Model file for the job. Use its own axes, mm. A direction names the side the tool comes from. Round coordinates to 2 decimals unless told otherwise and drop trailing zeros. Loops run counter-clockwise (first coordinate to the right, second up) from the corner with the lowest first, then second, coordinate; pieces in that order, holes last. Notation, with made-up numbers: (27, 59) -> (83, 59) arc R6 cw to (83, 67) -> close; hole circle Ø9 at (10.25, 39). An arc over 180 degrees is marked (long way). Use a Markdown table: item, result.
from build123d import *

# Parameters (mm, degrees)
F0_W      = 30
F0_H      = 22
F1_DEPTH  = 72
F3_DEPTH  = 72.001
F4_DEPTH  = 7
F6_DEPTH  = 7
F7_W      = 8
F7_H      = 44
F8_DEPTH  = 30.001
F9_W      = 30
F9_H      = 7
F10_DEPTH = 60
F11_R     = 4
F12_DEPTH = 65.001


with BuildPart() as f1:
    # F0 (on Top) → F1 (new body)
    with BuildSketch(Plane.XY):
        with Locations((15, 11)):
            Rectangle(F0_W, F0_H)
        Polygon((0, 102), (0, 22), (30, 22), (6.9943696583, 102.2807010551), align=None)
    extrude(amount=F1_DEPTH)

    # F2 (on face) → F3 (cut, through all)
    with BuildSketch(Plane.XY.offset(72)):
        Polygon((7, 22), (30, 22), (6.9943696583, 102.2807010551), align=None)
    extrude(amount=-F3_DEPTH, mode=Mode.SUBTRACT)

    # F2 (on face) → F4 (join)
    with BuildSketch(Plane.XY.offset(72)):
        Polygon((7, 22), (30, 22), (6.9943696583, 102.2807010551), align=None)
    extrude(amount=-F4_DEPTH)

    # F5 (on face) → F6 (join)
    with BuildSketch(Plane(origin=(0, 0, 0), x_dir=(1, 0, 0), z_dir=(0, 0, -1))):
        Polygon((6.9943696583, -102.2807010551), (30, -22), (7, -22), align=None)
    extrude(amount=-F6_DEPTH)

    # F7 (on face) → F8 (cut, through all)
    with BuildSketch(Plane.YZ.offset(30)):
        Polygon((16, 65), (8, 65), (8, 58), (8, 14), (8, 7), (16, 7), align=None)
        with Locations((4, 36)):
            Rectangle(F7_W, F7_H)
    extrude(amount=-F8_DEPTH, mode=Mode.SUBTRACT)

    # F9 (on face) → F10 (join)
    with BuildSketch(Plane.XZ):
        with Locations((15, 61.5)):
            Rectangle(F9_W, F9_H)
    extrude(amount=F10_DEPTH)

    # F11 (on face) → F12 (cut, through all)
    with BuildSketch(Plane.XY.offset(65)):
        with Locations((15, -44)):
            Circle(F11_R)
    extrude(amount=-F12_DEPTH, mode=Mode.SUBTRACT)


solid = f1.part
Q1. Band-saw the part on B-B, the plane x = 12.5. Give the cut face in (y, z), plus the area to 3 significant figures.
Results list:
| item | result |
|---|---|
| outline | (-60, 58) -> (-47.12, 58) -> (-47.12, 65) -> (-60, 65) -> close; (-40.88, 58) -> (8, 58) -> (8, 65) -> (16, 65) -> (16, 7) -> (8, 7) -> (8, 14) -> (0, 14) -> (0, 0) -> (83.07, 0) -> (83.07, 7) -> (22, 7) -> (22, 65) -> (83.07, 65) -> (83.07, 72) -> (0, 72) -> (0, 65) -> (-40.88, 65) -> close |
| area | 2,000 mm² |
Q2. Band-saw the part on D-D, the plane y = -44. Give the cut face in (x, z).
Results list:
| item | result |
|---|---|
| outline | (0, 58) -> (11, 58) -> (11, 65) -> (0, 65) -> close; (19, 58) -> (30, 58) -> (30, 65) -> (19, 65) -> close |
Q3. Band-saw the part on C-C, the plane z = 37. Give the cut face in (x, y), plus the area to 3 significant figures.
Results list:
| item | result |
|---|---|
| outline | (0, 16) -> (30, 16) -> (30, 22) -> (7, 22) -> (6.99, 102.28) -> (0, 102) -> close |
| area | 741 mm² |
Q4. Tool access for faces 1 (the face through (15, 4, 14)), 2 (the face through (15, -30, 65)), 3 (the face through (16, 53, 7)), 4 (the face through (15, 16, 36)): list every direction of +Z, -Z, +X, -X, +Y, -Y with a clear straight run to the whole face (end or side of a thin tool).
Results list:
| item | result |
|---|---|
| face 1 | +X, -X, -Y |
| face 2 | +Z, +X, -X, -Y |
| face 3 | +X, +Y |
| face 4 | +X, -X |
Q5. Band-saw the part on A-A, the plane y = 10. Give the cut face in (x, z), plus the area to 3 significant figures.
Results list:
| item | result |
|---|---|
| outline | (0, 0) -> (30, 0) -> (30, 7) -> (0, 7) -> close; (0, 65) -> (30, 65) -> (30, 72) -> (0, 72) -> close |
| area | 420 mm² |
Q6. Pull direction Y, two halves, no side cores. Call faces 5 (the face through (15, 12, 7)), 6 (the face through (18.658, 61.578, 68.549)), 7 (the face through (15, 8, 11)), 8 (the face through (11, 39, 0)): released by +Y, released by -Y, zero draft, split by the parting line, or undercut.
Results list:
| item | result |
|---|---|
| face 5 | undercut |
| face 6 | released by +Y |
| face 7 | undercut |
| face 8 | zero draft |
Q7. Drill centre lines: L1, parallel to Y at x = 15, z = 61.75; L2, parallel to Z at x = 25, y = 3; L3, parallel to Z at x = 25.5, y = -30. Where is each one in solid material? Low to high. Write a range as from..to.
Results list:
| item | result |
|---|---|
| L1 | y = -60..-48, -40..8, 16..22 |
| L2 | z = 0..14, 58..72 |
| L3 | z = 58..65 |
Q8. Flat gauge pins, fed straight in: pin 1 (10 mm diameter, centred on x = 18, y = -28.5, fed in from -Z); pin 2 (7 mm diameter, centred on x = 18, z = 49, fed in from +Y); pin 3 (7 mm diameter, centred on x = 11, z = 7, fed in from -Y). Where does each tip first touch, or does it go through?
Results list:
| item | result |
|---|---|
| pin 1 | stops at z = 58 |
| pin 2 | stops at y = 22 |
| pin 3 | stops at y = 0 |
